Could you check a few things on this drawing? It's one solid part, dimensions in mm from its lowest x, y, z. A direction names the side the tool comes from. Round coordinates to 2 decimals unless told otherwise and drop trailing zeros. Loops run counter-clockwise (first coordinate to the right, second up) from the corner with the lowest first, then second, coordinate; pieces in that order, holes last. Notation, with made-up numbers: M -6.5,-6.75 L 50.5,-6.75 A22 ccw 50.5,29.25 Z; hole C -13,41.25 d1. An arc over 180 degrees is marked long. Put each result on its own line as item: value. Start each with the question number.
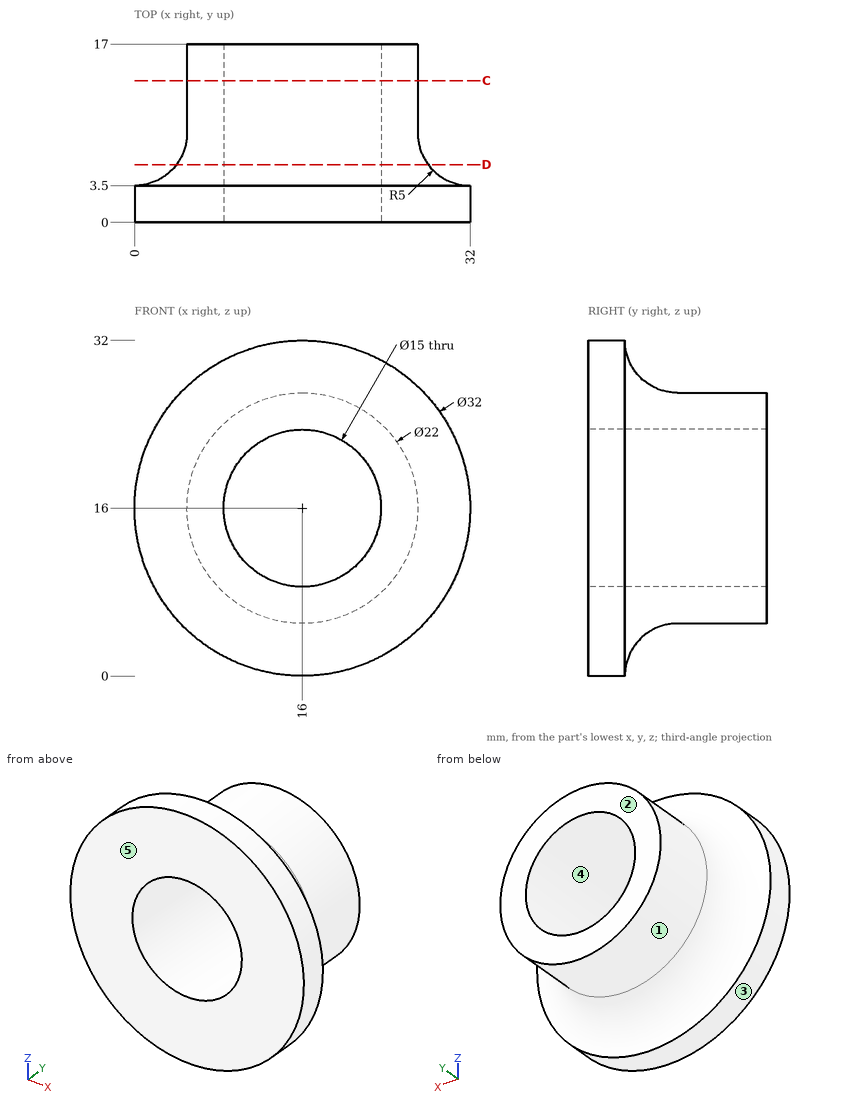
1) On a 3-axis mill with a long thin cutter (end or side, diameter ignored), from which of +Z, -Z, +X, -X, +Y, -Y can I reach the whole of each face in a straight line? I mean the marked faces 1 and 2. Say none if no direction works.
2) I'm going to push flat-ended pins straight in: P1, Ø4, axis at x = 26.5, z = 4.5, coming from the +Y side; P2, Ø1, axis at y = 2, z = 8, coming from the -X side; P3, Ø4, axis at y = 15, z = 24.5, coming from the +X side. Where does each tip first touch, or does it pass through?
3) Suppose I cut it at C-C (y = 13.5). Write out the boundary of the cut face in (x, z), plus the area to 3 significant figures.
4) Suppose I cut it at D-D (y = 5.5). Write out the boundary of the cut face in (x, z), plus the area to 3 significant figures.
5) If I drill on probe 1 along X at (y, z) = (11, 16); probe 2 along Z at (x, y) = (14.5, 8); probe 3 along Z at (x, y) = (20.5, 3), over which ranges is the centre line in solid material (lowest first)? Write a range as from..to.
6) If we mould it in two halves opening along X, with no side actions, what happens to the marked faces 3, 4 and 5? For each: pulls with the +X half, pulls with the -X half, needs draft (parallel to the pull), parting line crosses it, or undercut.
Results are:
1. face 1: +Y
1. face 2: +Z, -Z, +X, -X, +Y
2. P1: y = 4.13
2. P2: x = 1.87
2. P3: x = 24.87
3. outline: C 16,16 d22; hole C 16,16 d15
3. area: 203 mm²
4. outline: C 16,16 d24; hole C 16,16 d15
4. area: 276 mm²
5. probe 1: 5..8.5, 23.5..27
5. probe 2: 5.08..8.65, 23.35..26.92
5. probe 3: 0.65..10, 22..31.35
6. face 3: parting line crosses it
6. face 4: undercut
6. face 5: needs draft
